Check sheet for the modelled part. Datum: model origin and axes. Units: mm. Face numbers are marked on the shaded views. Round coordinates to 2 decimals unless told otherwise and drop trailing zeros. Loops run counter-clockwise (first coordinate to the right, second up) from the corner with the lowest first, then second, coordinate; pieces in that order, holes last. Notation, with made-up numbers: (89.5, 84) -> (117.5, 84) arc R10 cw to (117.5, 99) -> close; hole circle Ø2 at (28, 73.5). An arc over 180 degrees is marked (long way). Return JSON: item names as keys, results as strings.
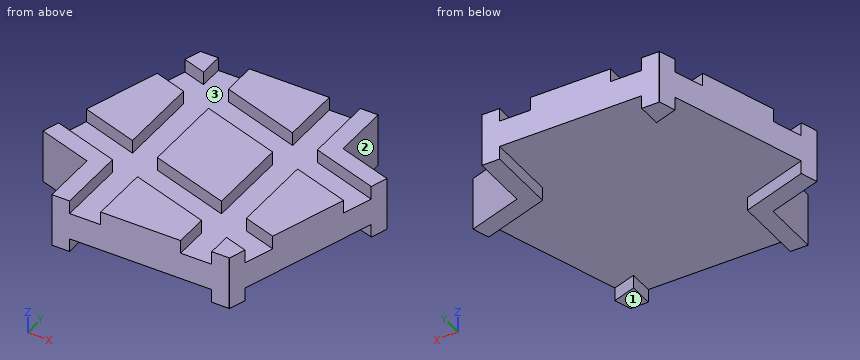
from build123d import *

# Parameters (mm, degrees)
SKETCH004_W = 32
SKETCH004_H = 3
SKETCH005_W = 7
SKETCH005_H = 3
SKETCH006_W = 7
SKETCH006_H = 3
SKETCH007_W = 32
SKETCH007_H = 3
SKETCH008_W = 7
SKETCH008_H = 3
SKETCH009_W = 7
SKETCH009_H = 3


with BuildPart() as part:
    # AdditivePipe: sweep along a path in Sketch
    with BuildLine(Plane.XY) as additivepipe_path:
        Line((0, -27.5), (0, 27.5))
    # Sketch002 (on DatumPlane) → AdditivePipe (sweep)
    with BuildSketch(Plane.XZ.offset(27.5)):
        Polygon((-20, 6), (-20, -6), (-16, -6), (-16, -3), (-9, -3), (9, -3), (16, -3), (16, -6), (20, -6), (20, 6), (16, 6), (16, 3), (9, 3), (9, 6), (-9, 6), (-9, 3), (-16, 3), (-16, 6), align=None)
    sweep(path=additivepipe_path.line)

    # AdditivePipe001: sweep along a path in Sketch001
    with BuildLine(Plane.XY) as additivepipe001_path:
        Line((-26.154054, 8.497967), (26.154054, -8.497967))
    # Sketch003 (on DatumPlane) → AdditivePipe001 (sweep)
    with BuildSketch(Plane(origin=(-26.154054, 8.497967, 0), x_dir=(-0.309017, -0.951057, 0), z_dir=(-0.951057, 0.309017, 0))):
        Polygon((-20, 6), (-20, -6), (-16, -6), (-16, -3), (-9, -3), (9, -3), (16, -3), (16, -6), (20, -6), (20, 6), (16, 6), (16, 3), (9, 3), (9, 6), (-9, 6), (-9, 3), (-16, 3), (-16, 6), align=None)
    sweep(path=additivepipe001_path.line)

    # SubtractivePipe: sweep along a path in Sketch
    with BuildLine(Plane.XY) as subtractivepipe_path:
        Line((0, -27.5), (0, 27.5))
    # Sketch004 (on DatumPlane) → SubtractivePipe (sweep, cut)
    with BuildSketch(Plane.XZ.offset(27.5)):
        with Locations((0, -4.5)):
            Rectangle(SKETCH004_W, SKETCH004_H)
    sweep(path=subtractivepipe_path.line, mode=Mode.SUBTRACT)

    # SubtractivePipe001: sweep along a path in Sketch
    with BuildLine(Plane.XY) as subtractivepipe001_path:
        Line((0, -27.5), (0, 27.5))
    # Sketch005 (on DatumPlane) → SubtractivePipe001 (sweep, cut)
    with BuildSketch(Plane.XZ.offset(27.5)):
        with Locations((-12.5, 4.5)):
            Rectangle(SKETCH005_W, SKETCH005_H)
    sweep(path=subtractivepipe001_path.line, mode=Mode.SUBTRACT)

    # SubtractivePipe002: sweep along a path in Sketch
    with BuildLine(Plane.XY) as subtractivepipe002_path:
        Line((0, -27.5), (0, 27.5))
    # Sketch006 (on DatumPlane) → SubtractivePipe002 (sweep, cut)
    with BuildSketch(Plane.XZ.offset(27.5)):
        with Locations((12.5, 4.5)):
            Rectangle(SKETCH006_W, SKETCH006_H)
    sweep(path=subtractivepipe002_path.line, mode=Mode.SUBTRACT)

    # SubtractivePipe003: sweep along a path in Sketch001
    with BuildLine(Plane.XY) as subtractivepipe003_path:
        Line((-26.154054, 8.497967), (26.154054, -8.497967))
    # Sketch007 (on DatumPlane) → SubtractivePipe003 (sweep, cut)
    with BuildSketch(Plane(origin=(-26.154054, 8.497967, 0), x_dir=(-0.309017, -0.951057, 0), z_dir=(-0.951057, 0.309017, 0))):
        with Locations((0, -4.5)):
            Rectangle(SKETCH007_W, SKETCH007_H)
    sweep(path=subtractivepipe003_path.line, mode=Mode.SUBTRACT)

    # SubtractivePipe004: sweep along a path in Sketch001
    with BuildLine(Plane.XY) as subtractivepipe004_path:
        Line((-26.154054, 8.497967), (26.154054, -8.497967))
    # Sketch008 (on DatumPlane) → SubtractivePipe004 (sweep, cut)
    with BuildSketch(Plane(origin=(-26.154054, 8.497967, 0), x_dir=(-0.309017, -0.951057, 0), z_dir=(-0.951057, 0.309017, 0))):
        with Locations((-12.5, 4.5)):
            Rectangle(SKETCH008_W, SKETCH008_H)
    sweep(path=subtractivepipe004_path.line, mode=Mode.SUBTRACT)

    # SubtractivePipe005: sweep along a path in Sketch001
    with BuildLine(Plane.XY) as subtractivepipe005_path:
        Line((-26.154054, 8.497967), (26.154054, -8.497967))
    # Sketch009 (on DatumPlane) → SubtractivePipe005 (sweep, cut)
    with BuildSketch(Plane(origin=(-26.154054, 8.497967, 0), x_dir=(-0.309017, -0.951057, 0), z_dir=(-0.951057, 0.309017, 0))):
        with Locations((12.5, 4.5)):
            Rectangle(SKETCH009_W, SKETCH009_H)
    sweep(path=subtractivepipe005_path.line, mode=Mode.SUBTRACT)


solid = part.part
Q1. Go/stop test with flat-tipped pins: pin 1 (1.5 mm diameter, centred on y = 23.5, z = -4.5, fed in from +X); pin 2 (4 mm diameter, centred on y = 1.5, z = -3, fed in from +X); pin 3 (0.9 mm diameter, centred on y = -25.5, z = -4, fed in from -X). Record where each tip stops, or that it passes through.
Results list:
{"pin 1": "x = 20", "pin 2": "x = 30.05", "pin 3": "x = -20"}
Q2. Draft check along X on the marked faces 1, 2 and 3. Enter one of: released by +X, released by -X, zero draft, split by the parting line, or undercut.
Results list:
{"face 1": "zero draft", "face 2": "released by +X", "face 3": "undercut"}
Q3. Section check D-D (x = 26). Record the boundary of the cut face in (y, z), then the cut area to 3 significant figures.
Results list:
{"outline": "(-8.97, -3) -> (8.38, -3) -> (8.38, -6) -> (12.58, -6) -> (12.58, 6) -> (8.38, 6) -> (8.38, 3) -> (1.02, 3) -> (1.02, 6) -> (-8.97, 6) -> close", "area": "185 mm^2"}
Q4. Section check C-C (x = 10). Record the boundary of the cut face in (y, z).
Results list:
{"outline": "(-27.5, -3) -> (27.5, -3) -> (27.5, 3) -> (-27.5, 3) -> close"}
Q5. Material ranges on line 1 (Y direction, x = 1, z = 5.5); line 2 (Z direction, x = -5.5, y = 17); line 3 (Z direction, x = 17.5, y = -12), recorded low to high.
Results list:
{"line 1": "-27.5 to -17.15, -9.79 to 9.14, 16.5 to 27.5", "line 2": "-3 to 3", "line 3": "-3 to 6"}
Q6. Section check B-B (y = -2). Record the boundary of the cut face in (x, z).
Results list:
{"outline": "(-29.57, -3) -> (28.27, -3) -> (28.27, 6) -> (16, 6) -> (16, 3) -> (9, 3) -> (9, 6) -> (-9, 6) -> (-9, 3) -> (-16, 3) -> (-16, 6) -> (-22.97, 6) -> (-22.97, 3) -> (-29.57, 3) -> close"}
